The listing builds one solid part. Answer for the finished solid, in the listing's coordinates (mm). Face numbers are marked on the shaded views. A direction names the side the tool comes from. Give positions to 0.01 mm unless a question says otherwise; leave off trailing zeros. Write each loop counter-clockwise with the first axis right and the second up, starting at its lowest first coordinate (ties: lowest second). Pieces come first, ordered by that corner, then holes.
```python
from build123d import *

# Parameters (mm, degrees)
SKETCH1_R           = 2.29235
BOSS_EXTRUDE1_DEPTH = 6.35


with BuildPart() as part:
    # Sketch1 → Boss-Extrude1 (new body)
    with BuildSketch(Plane(origin=(0, 0, 0), x_dir=(1, 0, 0), z_dir=(0, 1, 0))):
        with BuildLine():
            Line((0.048227533, 4.445), (32.250386453, 4.445))
            ThreePointArc((32.250386453, 4.445), (33.423227931, 4.731992484), (34.331032646, 5.528115852))
            Line((34.331032646, 5.528115852), (49.159221832, 26.704964681))
            Line((49.159221832, 26.704964681), (49.900908924, 29.244964681))
            ThreePointArc((49.900908924, 29.244964681), (55.562425443, 32.347386681), (58.664847444, 26.685870162))
            Line((58.664847444, 26.685870162), (56.441483505, 21.605870162))
            Line((56.441483505, 21.605870162), (38.958873725, -3.361884148))
            ThreePointArc((38.958873725, -3.361884148), (38.05106901, -4.158007516), (36.878227533, -4.445))
            Line((36.878227533, -4.445), (0.048227533, -4.445))
            ThreePointArc((0.048227533, -4.445), (-4.445261623, 0), (0.048227533, 4.445))
        make_face()
        Circle(SKETCH1_R, mode=Mode.SUBTRACT)
        with Locations((35.737148471, 0.286992484)):
            Circle(SKETCH1_R, mode=Mode.SUBTRACT)
        with Locations((54.282878184, 27.965417421)):
            Circle(SKETCH1_R, mode=Mode.SUBTRACT)
    extrude(amount=BOSS_EXTRUDE1_DEPTH)


solid = part.part
```
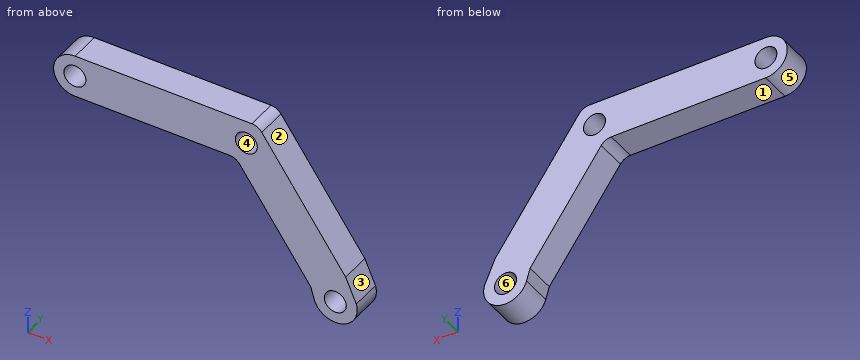
Item 1: Each of these flat-tipped pins is pushed along its axis until it touches: P1, Ø3.5, axis at x = 0, z = 0, coming from the +Y side; P2, Ø8, axis at x = 51, z = -11.5, coming from the +Y side; P3, Ø2, axis at y = 1.5, z = -8.5, coming from the -X side; P4, Ø3, axis at x = 32, y = 4, coming from the -Z side. Where does it stop, or does it pass through?
Conclusion:
P1: passes through
P2: stops at y = 6.35
P3: stops at x = 35.71
P4: stops at z = -4.77
Item 2: Which of the six approach directions +Z, -Z, +X, -X, +Y, -Y give full straight-line access (tool end or side, diameter ignored) to the marked faces 1 and 2?
Conclusion:
face 1: -Z, -X, +Y, -Y
face 2: +Z, +X, +Y, -Y
Item 3: A cutting plane is placed at D-D, the plane z = -23.5. Give the vertices of the cut face in (x, y), plus the area to 3 significant figures.
Conclusion:
outline: (46.92, 0) - (57.27, 0) - (57.27, 6.35) - (46.92, 6.35) - close
area: 65.8 mm2
Item 4: A cutting plane is placed at B-B, the plane y = 1.25. Give the vertices of the cut face in (x, z) (1 decimal), plus the area to 3 significant figures.
Conclusion:
outline: (0, -4.4) - (32.3, -4.4) arc R2.5 cw to (34.3, -5.5) - (49.2, -26.7) - (49.9, -29.2) arc R4.6 ccw to (58.7, -26.7) - (56.4, -21.6) - (39, 3.4) arc R2.5 ccw to (36.9, 4.4) - (0, 4.4) arc R4.4 ccw (long way) to start; hole circle Ø4.6 at (0, 0); hole circle Ø4.6 at (35.7, -0.3); hole circle Ø4.6 at (54.3, -28)
area: 632 mm2
Item 5: Determine the mould class of the marked faces 3, 4, 5 and 6 for opening direction Z: pulls with the +Z half, pulls with the -Z half, needs draft (parallel to the pull), parting line crosses it, or undercut.
Conclusion:
face 3: pulls with the +Z half
face 4: undercut
face 5: parting line crosses it
face 6: undercut
Item 6: Consider probe 1 along Z at (x, y) = (0, 4.25); probe 2 along Z at (x, y) = (4.5, 1.25) (3 decimals); probe 3 along X at (y, z) = (3.75, -2). Determine where each line is inside the solid, lowest interval first.
Conclusion:
probe 1: z = -4.45 to -2.29, 2.29 to 4.45
probe 2: z = -4.445 to 4.445
probe 3: x = -3.97 to -1.12, 1.12 to 34.21, 37.26 to 42.71
Item 7: A cutting plane is placed at A-A, the plane z = -1. Give the vertices of the cut face in (x, y), plus the area to 3 significant figures.
Conclusion:
outline: (-4.33, 0) - (-2.06, 0) - (-2.06, 6.35) - (-4.33, 6.35) - close; (2.06, 0) - (33.56, 0) - (33.56, 6.35) - (2.06, 6.35) - close; (37.92, 0) - (42.01, 0) - (42.01, 6.35) - (37.92, 6.35) - close
area: 240 mm2
Item 8: A cutting plane is placed at C-C, the plane x = 31.5. Give the vertices of the cut face in (y, z) (3 decimals).
Conclusion:
outline: (0, -4.445) - (6.35, -4.445) - (6.35, 4.445) - (0, 4.445) - close
